Model file for the job. Use its own axes, mm. Face numbers are marked on the shaded views. A direction names the side the tool comes from. Give positions to 0.01 mm unless a question says otherwise; leave off trailing zeros. Answer in a Markdown table with one row per item.
```python
from build123d import *

# Parameters (mm, degrees)
EXTRUDE_1_DEPTH     = 10
FILLET_5_R          = 5
FILLET_6_R          = 5
SKETCH_22_R         = 2.8
CUT_EXTRUDE_1_DEPTH = 3.4


with BuildPart() as part:
    # Эскиз2 → Бобышка-Вытянуть1 (new body)
    with BuildSketch(Plane(origin=(0, 0, 0), x_dir=(1, 0, 0), z_dir=(0, 1, 0))):
        with BuildLine():
            Line((10, -25), (20, -20))
            ThreePointArc((20, -20), (30, -10), (20, 0))
            Line((20, 0), (0, 0))
            Line((0, 0), (-17.215189328, -10.180238524))
            Line((-17.215189328, -10.180238524), (-32.215189328, -10.180238524))
            Line((-32.215189328, -10.180238524), (-32.215189328, -0.180238524))
            Line((-32.215189328, -0.180238524), (-17.215189328, -0.180238524))
            Line((-17.215189328, -0.180238524), (0, 10))
            Line((0, 10), (20, 10))
            ThreePointArc((20, 10), (40, -10), (20, -30))
            Line((20, -30), (10, -25))
        make_face()
    extrude(amount=EXTRUDE_1_DEPTH)

    # Скругление5
    fillet_5_edges = [part.edges().sort_by_distance(p)[0] for p in [
        (30, 10, 10),
        (30, 0, 10),
        (10, 10, 0),
        (10, 0, 0),
        (-24.715189328, 10, 10.180238524),
        (-24.715189328, 0, 10.180238524),
    ]]
    fillet(fillet_5_edges, radius=FILLET_5_R - 0.0001)  # a hair under: the kernel refuses the full size

    # Скругление6
    fillet_6_edges = [part.edges().sort_by_distance(p)[0] for p in [
        (40, 10, 10),
        (40, 0, 10),
        (10, 10, -10),
        (10, 0, -10),
        (-8.607594664, 10, -4.909880738),
        (-8.607594664, 0, -4.909880738),
        (-24.715189328, 10, 0.180238524),
        (-24.715189328, 0, 0.180238524),
    ]]
    fillet(fillet_6_edges, radius=FILLET_6_R - 0.0001)  # a hair under: the kernel refuses the full size

    # Эскиз22 → Вырез-Вытянуть1 (cut)
    with BuildSketch(Plane.ZY.offset(32.215189328)):
        with Locations((5.180238524, 5)):
            Circle(SKETCH_22_R)
    extrude(amount=-CUT_EXTRUDE_1_DEPTH, mode=Mode.SUBTRACT)


solid = part.part
```
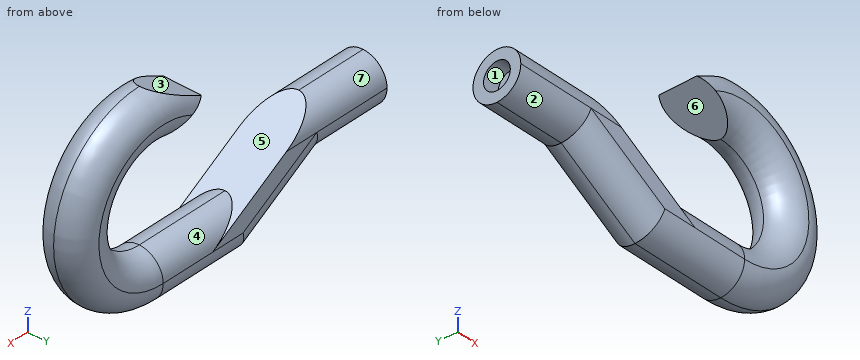
Q1. Drop flat-ended pins along their axis: pin 1 (1.5 mm diameter, centred on x = -3, y = 8.5, fed in from -Z); pin 2 (1.5 mm diameter, centred on x = 22, z = 23, fed in from +Y); pin 3 (4.5 mm diameter, centred on y = 6, z = 5, fed in from -X); pin 4 (4 mm diameter, centred on x = -22, y = 3, fed in from -Z). Give the stop position or say it passes through.
Reported:
| item | result |
|---|---|
| pin 1 | z = -7.42 |
| pin 2 | y = 9.88 |
| pin 3 | x = -32.22 |
| pin 4 | z = 0.18 |
Q2. Probe probe 1 along X at (y, z) = (7.5, 2.5); probe 2 along X at (y, z) = (8.5, 0); probe 3 along X at (y, z) = (2, 24). List the from-to ranges inside material, lowest first.
Reported:
| item | result |
|---|---|
| probe 1 | -32.22 to -4.23, 27.59 to 37.82 |
| probe 2 | -14.1 to 0, 25.53 to 35.65 |
| probe 3 | 12 to 32.85 |
Q3. 3-axis set-ups, long thin cutter, end or side, ignore diameter. For the marked faces 1, 2, 3 and 4: which of +Z, -Z, +X, -X, +Y, -Y reach the whole face in a straight line?
Reported:
| item | result |
|---|---|
| face 1 | -X |
| face 2 | -Z, -X, -Y |
| face 3 | +Z, -X, +Y, -Y |
| face 4 | +Y |
Q4. Mould opens along X. For the marked faces 5, 6 and 7 say: released by +X, released by -X, zero draft, split by the parting line, or undercut.
Reported:
| item | result |
|---|---|
| face 5 | undercut |
| face 6 | released by -X |
| face 7 | zero draft |
